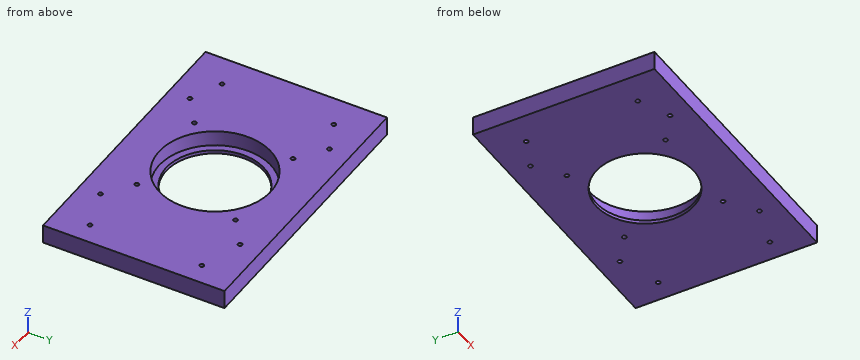
from build123d import *

# Parameters (mm, degrees)
SKETCH_W     = 200
SKETCH_H     = 130
SKETCH_R     = 35
SKETCH_R_2   = 1.5
PAD_DEPTH    = 13.5
SKETCH001_R  = 40
POCKET_DEPTH = 11


with BuildPart() as part:
    # Sketch → Pad (new body)
    with BuildSketch(Plane.XY):
        with Locations((100, 65)):
            Rectangle(SKETCH_W, SKETCH_H)
        with Locations((100, 65)):
            Circle(SKETCH_R, mode=Mode.SUBTRACT)
        with Locations((45, 115)):
            Circle(SKETCH_R_2, mode=Mode.SUBTRACT)
        with Locations((45, 15)):
            Circle(SKETCH_R_2, mode=Mode.SUBTRACT)
        with Locations((155, 115)):
            Circle(SKETCH_R_2, mode=Mode.SUBTRACT)
        with Locations((155, 15)):
            Circle(SKETCH_R_2, mode=Mode.SUBTRACT)
        with Locations((22.5, 105)):
            Circle(SKETCH_R_2, mode=Mode.SUBTRACT)
        with Locations((22.5, 25)):
            Circle(SKETCH_R_2, mode=Mode.SUBTRACT)
        with Locations((185, 105)):
            Circle(SKETCH_R_2, mode=Mode.SUBTRACT)
        with Locations((185, 25)):
            Circle(SKETCH_R_2, mode=Mode.SUBTRACT)
        with Locations((135.350164, 100.350164)):
            Circle(SKETCH_R_2, mode=Mode.SUBTRACT)
        with Locations((64.639486, 29.639486)):
            Circle(SKETCH_R_2, mode=Mode.SUBTRACT)
        with Locations((64.64463, 100.35537)):
            Circle(SKETCH_R_2, mode=Mode.SUBTRACT)
        with Locations((135.359088, 29.640912)):
            Circle(SKETCH_R_2, mode=Mode.SUBTRACT)
    extrude(amount=PAD_DEPTH)

    # Sketch001 (on Face19 of Pad) → Pocket (cut)
    with BuildSketch(Plane.XY.offset(13.5)):
        with Locations((100, 65)):
            Circle(SKETCH001_R)
    extrude(amount=-POCKET_DEPTH, mode=Mode.SUBTRACT)


solid = part.part
Input: part model. Units: mm. Frame: model coordinates. Round coordinates to 2 decimals unless told otherwise and drop trailing zeros. Order: outer loops, then holes, each group sorted by start corner. A loop starts at its lowest first (then second) coordinate and runs counter-clockwise, first axis right, second up.
1. Cut plane A-A, the plane x = 100. Output: boundary loops of the cut face in (y, z), then the cut area to 3 significant figures.
The answers:
outline: (0, 0) - (30, 0) - (30, 2.5) - (25, 2.5) - (25, 13.5) - (0, 13.5) - close; (100, 0) - (130, 0) - (130, 13.5) - (105, 13.5) - (105, 2.5) - (100, 2.5) - close
area: 700 mm2
2. Material intervals for line 1 (X direction, y = 105, z = 2.25); line 2 (Y direction, x = 45, z = 4); line 3 (Y direction, x = 109.5, z = 8), sorted ascending.
The answers:
line 1: x = 0 to 21, 24 to 183.5, 186.5 to 200
line 2: y = 0 to 13.5, 16.5 to 113.5, 116.5 to 130
line 3: y = 0 to 26.14, 103.86 to 130
3. Cut plane C-C, the plane z = 9.5. State how many separate pieces and enclosed holes the cut face has, then the cut area to 3 significant figures.
The answers:
separate pieces: 1
enclosed holes: 13
area: 20,900 mm2
4. Pin query (flat end, axial travel): P1, Ø5, axis at x = 135.35, y = 100.35, coming from the -Z side. Return the tip coordinate at first contact, or that it passes through.
The answers:
P1: stops at z = 0
5. Cut plane B-B, the plane y = 65. Output: boundary loops of the cut face in (x, z).
The answers:
outline: (0, 0) - (65, 0) - (65, 2.5) - (60, 2.5) - (60, 13.5) - (0, 13.5) - close; (135, 0) - (200, 0) - (200, 13.5) - (140, 13.5) - (140, 2.5) - (135, 2.5) - close
